Source: CAD feature listing. Evaluate the final solid. Frame: model axes, mm. Face numbers are marked on the shaded views. A direction names the side the tool comes from. Give positions to 0.01 mm unless a question says otherwise; leave off trailing zeros. Write each loop counter-clockwise with the first axis right and the second up, starting at its lowest first coordinate (ties: lowest second). Pieces come first, ordered by that corner, then holes. Notation, with made-up numbers: (-18, 48.5) -> (2, 48.5) arc R21 cw to (2, 67.5) -> close; hole circle Ø5 at (39, -9.75). An arc over 180 degrees is marked (long way). Answer as a JSON object with one key per item and string values. Group by question number.
Item 1: First-contact query: pin 1 Ø6 at (x, y) = (105, 59.5) entering from -Z; pin 2 Ø12 at (y, z) = (36.5, -24) entering from +X; pin 3 Ø4 at (y, z) = (26.5, -122.5) entering from -X. Flat tips, straight axial feed; report the tip coordinate or a pass-through.
Item 2: Section query C-C on y = 33. Return the cut outline in (x, z), plus the area to 3 significant figures.
Item 3: Ray query, probe 1 along Z at (x, y) = (348, 1.5); probe 2 along Z at (x, y) = (-182, -82.5); probe 3 along X at (y, z) = (38, -34). Return the intervals inside material, ascending. Write a range as from..to.
Item 4: Pull-direction query (Z, two-part tool) for the marked faces 3, 4 and 5; classes: pulls with the +Z half, pulls with the -Z half, needs draft (parallel to the pull), parting line crosses it, or undercut.
Item 5: Access query for the marked faces 1 and 2. Directions: +Z, -Z, +X, -X, +Y, -Y. A direction counts if a zero-diameter tool reaches every point of the face in a straight line with its end or side. Return the directions, or none.
Item 6: Section query A-A on x = -290. Return the cut outline in (y, z).
Item 7: Section query D-D on y = -8.5. Return the cut outline in (x, z).
Item 8: Section query B-B on z = -85. Return the cut outline in (x, y), plus the area to 3 significant figures.
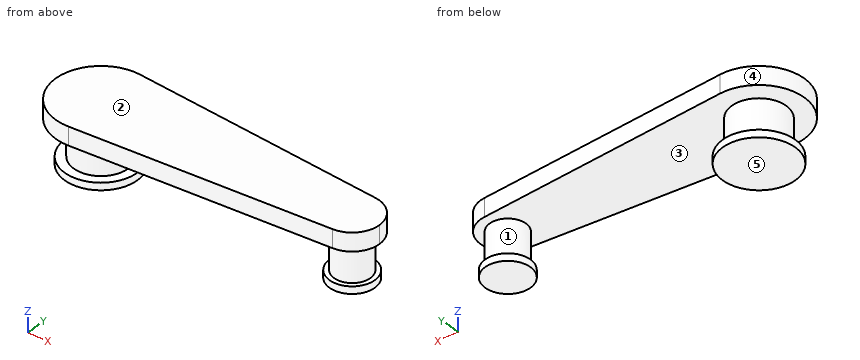
from build123d import *

# Parameters (mm, degrees)
BOSS_EXTRUDE1_DEPTH = 25
SKETCH2_R           = 75
SKETCH2_R_2         = 50
BOSS_EXTRUDE2_DEPTH = 100
SKETCH3_R           = 62.5
SKETCH3_R_2         = 100
BOSS_EXTRUDE3_DEPTH = 20


with BuildPart() as part:
    # Sketch1 → Boss-Extrude1 (new, symmetric)
    with BuildSketch(Plane.XY):
        with BuildLine():
            ThreePointArc((-215, 0), (-290, 75), (-365, 0))
            Line((-365, 0), (-215, 0))
        make_face()
        with BuildLine():
            Line((-215, 0), (-365, 0))
            ThreePointArc((-365, 0), (-290, -75), (-215, 0))
        make_face()
        with BuildLine():
            Line((405.434782609, 74.802828409), (-280.942028986, 124.671380682))
            ThreePointArc((-280.942028986, 124.671380682), (-375.125653076, 91.534819541), (-415, 0))
            Line((-415, 0), (-365, 0))
            ThreePointArc((-365, 0), (-290, 75), (-215, 0))
            Line((-215, 0), (350, 0))
            ThreePointArc((350, 0), (400, 50), (450, 0))
            Line((450, 0), (475, 0))
            ThreePointArc((475, 0), (454.920891725, 51.075391846), (405.434782609, 74.802828409))
        make_face()
        with BuildLine():
            Line((-365, 0), (-415, 0))
            ThreePointArc((-415, 0), (-375.125653076, -91.534819541), (-280.942028986, -124.671380682))
            Line((-280.942028986, -124.671380682), (405.434782609, -74.802828409))
            ThreePointArc((405.434782609, -74.802828409), (454.920891725, -51.075391846), (475, 0))
            Line((475, 0), (450, 0))
            ThreePointArc((450, 0), (400, -50), (350, 0))
            Line((350, 0), (-215, 0))
            ThreePointArc((-215, 0), (-290, -75), (-365, 0))
        make_face()
        with BuildLine():
            ThreePointArc((350, 0), (400, -50), (450, 0))
            Line((450, 0), (350, 0))
        make_face()
        with BuildLine():
            Line((350, 0), (450, 0))
            ThreePointArc((450, 0), (400, 50), (350, 0))
        make_face()
    extrude(amount=BOSS_EXTRUDE1_DEPTH, both=True)

    # Sketch2 → Boss-Extrude2 (add)
    with BuildSketch(Plane(origin=(0, 0, -25), x_dir=(-1, 0, 0), z_dir=(0, 0, -1))):
        with Locations(Location((290, 0, 0), (0, 0, 180))):
            Circle(SKETCH2_R)
        with Locations(Location((-400, 0, 0), (0, 0, 180))):
            Circle(SKETCH2_R_2)
    extrude(amount=BOSS_EXTRUDE2_DEPTH)

    # Sketch3 → Boss-Extrude3 (add)
    with BuildSketch(Plane(origin=(0, 0, -125), x_dir=(-1, 0, 0), z_dir=(0, 0, -1))):
        with Locations((-400, 0)):
            Circle(SKETCH3_R)
        with Locations((290, 0)):
            Circle(SKETCH3_R_2)
    extrude(amount=BOSS_EXTRUDE3_DEPTH)


solid = part.part
Worked answers:
{
 "1": {"pin 1": "z = -25", "pin 2": "x = 468.52", "pin 3": "x = -360.89"},
 "2": {"outline": "(-410.57, -25) -> (-357.35, -25) -> (-357.35, -125) -> (-384.4, -125) -> (-384.4, -145) -> (-195.6, -145) -> (-195.6, -125) -> (-222.65, -125) -> (-222.65, -25) -> (362.44, -25) -> (362.44, -125) -> (346.92, -125) -> (346.92, -145) -> (453.08, -145) -> (453.08, -125) -> (437.56, -125) -> (437.56, -25) -> (467.35, -25) -> (467.35, 25) -> (-410.57, 25) -> close", "area": "70,800 mm^2"},
 "3": {"probe 1": "-145..-125, -25..25", "probe 2": "-25..25", "probe 3": "-354.66..-225.34, 367.5..432.5"},
 "4": {"face 3": "undercut", "face 4": "needs draft", "face 5": "pulls with the -Z half"},
 "5": {"face 1": "none", "face 2": "+Z, +X, -X, +Y, -Y"},
 "6": {"outline": "(-125, -25) -> (-75, -25) -> (-75, -125) -> (-100, -125) -> (-100, -145) -> (100, -145) -> (100, -125) -> (75, -125) -> (75, -25) -> (125, -25) -> (125, 25) -> (-125, 25) -> close"},
 "7": {"outline": "(-414.71, -25) -> (-364.52, -25) -> (-364.52, -125) -> (-389.64, -125) -> (-389.64, -145) -> (-190.36, -145) -> (-190.36, -125) -> (-215.48, -125) -> (-215.48, -25) -> (350.73, -25) -> (350.73, -125) -> (338.08, -125) -> (338.08, -145) -> (461.92, -145) -> (461.92, -125) -> (449.27, -125) -> (449.27, -25) -> (474.52, -25) -> (474.52, 25) -> (-414.71, 25) -> close"},
 "8": {"outline": "circle Ø150 at (-290, 0); circle Ø100 at (400, 0)", "area": "25,500 mm^2"}
}
